Check sheet for the drawn part. Datum: minimum x, y, z corner. Units: mm. Give positions to 0.01 mm unless a question says otherwise; leave off trailing zeros. Write each loop counter-clockwise with the first axis right and the second up, starting at its lowest first coordinate (ties: lowest second). Pieces come first, ordered by that corner, then holes.
(1) Cross-section at C-C (z = 1.5). Record the boundary of the cut face in (x, y).
(2) Depth check by flat-ended pin: P1, Ø3, axis at y = 61.5, z = 2.5, coming from the +X side. Enter the tip coordinate at first touch or a pass-through.
(3) Cross-section at B-B (y = 86). Record the boundary of the cut face in (x, z), and give its area (3 significant figures).
(4) Cross-section at A-A (x = 43). Record the boundary of the cut face in (y, z), and give its area (3 significant figures).
(5) Thickness scan on line 1 along X through (y, z) = (214.5, 2.75) (3 decimals); line 2 along X through (y, z) = (262, 2). Record the ranges inside material, lowest first.
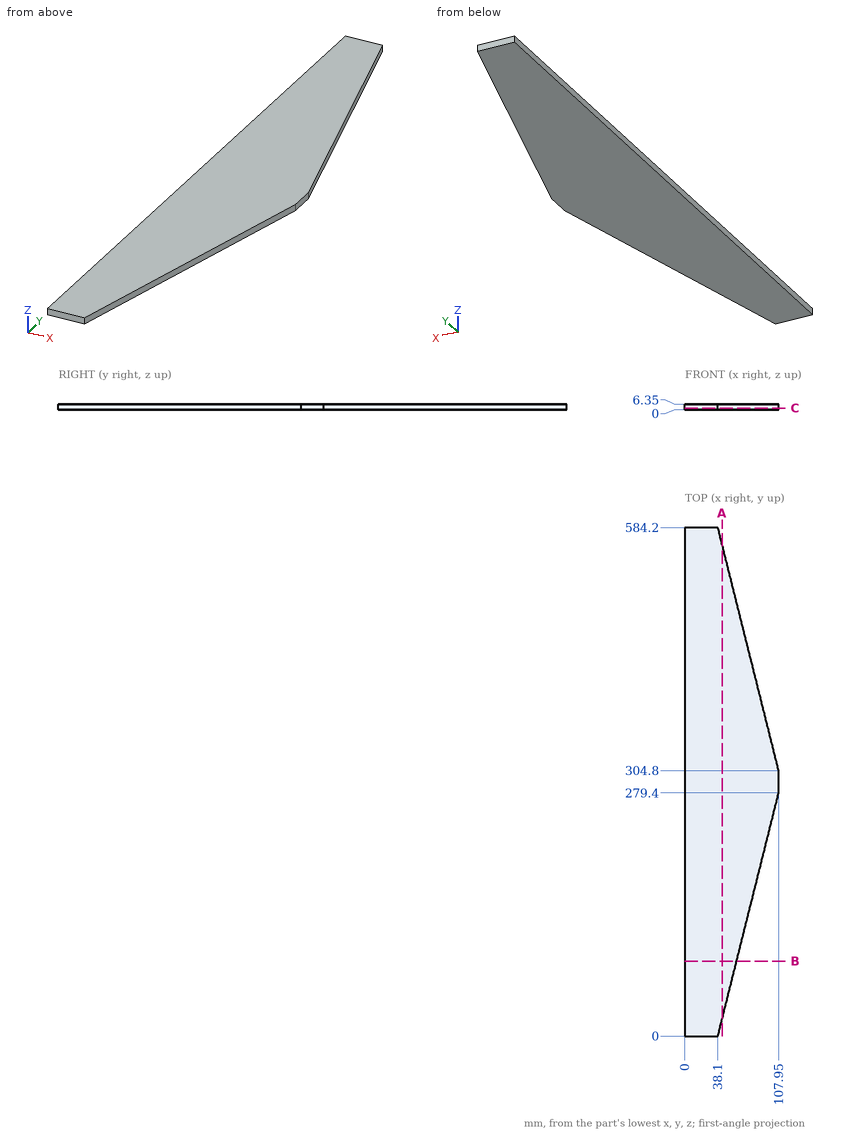
Reply:
1. outline: (0, 0) - (38.1, 0) - (107.95, 279.4) - (107.95, 304.8) - (38.1, 584.2) - (0, 584.2) - close
2. P1: stops at x = 53.85
3. outline: (0, 0) - (59.6, 0) - (59.6, 6.35) - (0, 6.35) - close
3. area: 378 mm2
4. outline: (19.6, 0) - (564.6, 0) - (564.6, 6.35) - (19.6, 6.35) - close
4. area: 3,460 mm2
5. line 1: x = 0 to 91.725
5. line 2: x = 0 to 103.6
